Work out the finished part from the listing and answer in its coordinate system (mm). A direction names the side the tool comes from. Give positions to 0.01 mm unless a question says otherwise; leave off trailing zeros. Loops run counter-clockwise (first coordinate to the right, second up) from the corner with the lowest first, then second, coordinate; pieces in that order, holes last. Notation, with made-up numbers: (16.5, 57) -> (24.5, 57) arc R26 cw to (24.5, 89) -> close; hole circle Ø3 at (-5, 20). An arc over 180 degrees is marked (long way). Answer as CSV lines item,"result". Start each with the question number.
1. Find section D-D, the plane x = 73. Give the vertices of the cut face in (y, z) (3 decimals), and give its area (3 significant figures).
2. Find the intervals of material crossed by line 1 along Y through (x, z) = (39.5, 30.5); line 2 along X through (y, z) = (1.5, 64); line 3 along Z through (x, y) = (21, 48.5) (3 decimals), in increasing order.
3. A tool of negligible diameter and unlimited length cuts with its end or side. For faces 1 (the face through (22.225, 17, 18)), 2 (the face through (79, -1, 38.1)), 3 (the face through (-1, -7.938, 30)), 4 (the face through (-1, -1, -9.525)), 5 (the face through (-39.464, 61.59, -0.133)), from which of +Z, -Z, +X, -X, +Y, -Y can it reach the whole face along a straight path? Write none if from no direction.
4. Find section A-A, the plane z = -4. Give the vertices of the cut face in (x, y) (3 decimals), and give its area (3 significant figures).
5. Flat-ended cylindrical pins translate along their axes: pin 1 Ø4 at (x, z) = (39.5, 13) entering from -Y; pin 2 Ø15 at (x, z) = (4, 36.5) entering from -Y; pin 3 Ø4 at (x, y) = (75.5, 36.5) entering from -Z; pin 4 Ø19 at (y, z) = (14, 17.5) entering from -X (3 decimals). Find the tip coordinate at first contact, or state that the pin passes through.
6. Find section C-C, the plane x = 90. Give the vertices of the cut face in (y, z) (3 decimals).
7. Find section B-B, the plane y = 14.5. Give the vertices of the cut face in (x, z) (3 decimals).
from build123d import *

# Parameters (mm, degrees)
F1_DEPTH = 63.5
F2_DEPTH = 25.4
F3_DEPTH = 7.9375
F0_W     = 37.164882
F0_H     = 28.575
F5_R     = 6.35


with BuildPart() as f1:
    # F0 (on Front) → F1 (new body, symmetric)
    with BuildSketch(Plane.XZ):
        Polygon((-41.275, 9.525), (-41.275, -9.525), (41.275, -9.525), (41.275, 9.525), (22.225, 9.525), align=None)
    extrude(amount=F1_DEPTH, both=True)

    # F0 (on Front) → F2 (join, symmetric)
    with BuildSketch(Plane.XZ):
        with BuildLine():
            Line((22.225, 9.525), (41.275, 9.525))
            Line((41.275, 9.525), (41.275, 27.0002))
            ThreePointArc((41.275, 27.0002), (45.92468, 38.22552), (57.15, 42.8752))
            Line((57.15, 42.8752), (60.325, 42.8752))
            Line((60.325, 42.8752), (60.325, 61.9252))
            Line((60.325, 61.9252), (57.15, 61.9252))
            ThreePointArc((57.15, 61.9252), (32.454296, 51.695904), (22.225, 27.0002))
            Line((22.225, 27.0002), (22.225, 9.525))
        make_face()
        Polygon((60.325, 66.675), (60.325, 61.9252), (60.325, 42.8752), (60.325, 38.1), (73.960118, 38.1), (73.960118, 66.675), align=None)
    extrude(amount=F2_DEPTH, both=True)

    # F0 (on Front) → F3 (join, symmetric)
    with BuildSketch(Plane.XZ):
        with BuildLine():
            add(Edge.make_bspline(
                [(-41.275, 9.525), (-30.2571, 34.45055), (20.033766, 63.231468), (57.15, 61.9252)],
                knots=[0, 0, 0, 0, 111.504536, 111.504536, 111.504536, 111.504536], degree=3))
            Line((-41.275, 9.525), (22.225, 9.525))
            Line((22.225, 9.525), (22.225, 27.0002))
            ThreePointArc((22.225, 27.0002), (32.454296, 51.695904), (57.15, 61.9252))
        make_face()
    extrude(amount=F3_DEPTH, both=True)

    # F0 (on Front) → F4 (revolve)
    with BuildSketch(Plane.XZ):
        with Locations((92.542559, 52.3875)):
            Rectangle(F0_W, F0_H)
    revolve(axis=Axis((73.960118, 0, 52.3875), (0, 0, -1)))

    # F5
    f5_edges = [f1.edges().sort_by_distance(p)[0] for p in [
        (-41.275, -63.5, 0),
        (41.275, -63.5, 0),
        (-41.275, 63.5, 0),
        (41.275, 63.5, 0),
    ]]
    fillet(f5_edges, radius=F5_R)


solid = f1.part
Resolved:
1,outline,"(-37.152, 38.1) -> (37.152, 38.1) -> (37.152, 66.675) -> (-37.152, 66.675) -> close"
1,area,"2,120 mm^2"
2,line 1,"y = -25.4 to 25.4"
2,line 2,"x = 36.83 to 111.09"
2,line 3,"z = -9.525 to 9.525"
3,face 1,"+Z, -X, +Y"
3,face 2,"-Z, +X, +Y, -Y"
3,face 3,"+Z, -X, -Y"
3,face 4,"-Z, +X, -X, +Y, -Y"
3,face 5,"+Z, -Z, -X, +Y"
4,outline,"(-41.275, -57.15) arc R6.35 ccw to (-34.925, -63.5) -> (34.925, -63.5) arc R6.35 ccw to (41.275, -57.15) -> (41.275, 57.15) arc R6.35 ccw to (34.925, 63.5) -> (-34.925, 63.5) arc R6.35 ccw to (-41.275, 57.15) -> close"
4,area,"10,400 mm^2"
5,pin 1,"stops at y = -25.4"
5,pin 2,"stops at y = -7.94"
5,pin 3,"stops at z = 38.1"
5,pin 4,"stops at x = -41.275"
6,outline,"(-33.525, 38.1) -> (33.525, 38.1) -> (33.525, 66.675) -> (-33.525, 66.675) -> close"
7,outline,"(-41.275, -9.525) -> (41.275, -9.525) -> (41.275, 27) arc R15.875 cw to (45.801, 38.1) -> (108.18, 38.1) -> (108.18, 66.675) -> (39.741, 66.675) -> (39.741, 57.277) arc R34.925 ccw to (22.225, 27) -> (22.225, 9.525) -> (-41.275, 9.525) -> close"
